```python
from build123d import *

# Parameters (mm, degrees)
SKETCH_1_W               = 20
SKETCH_1_H               = 20
SKETCH_1_R               = 2
SKETCH_1_R_2             = 2.15
EXTRUDE_1_DEPTH          = 46
CUT_EXTRUDE_1_REACH      = 50.125
PATTERN_CIRCULAR_1_COUNT = 4
FILLET_1_R               = 0.3
CUT_EXTRUDE_2_DEPTH      = 49.124837662
CUT_EXTRUDE_2_DEPTH_BACK = 49.124837662
SKETCH_2_R               = 2.5


with BuildPart() as part:
    # Sketch 1 → Extrude 1 (new body)
    with BuildSketch(Plane.XY):
        Rectangle(SKETCH_1_W, SKETCH_1_H)
        with Locations((-7, 7)):
            Circle(SKETCH_1_R, mode=Mode.SUBTRACT)
        with Locations((-7, -7)):
            Circle(SKETCH_1_R, mode=Mode.SUBTRACT)
        Circle(SKETCH_1_R_2, mode=Mode.SUBTRACT)
        with Locations((7, 7)):
            Circle(SKETCH_1_R, mode=Mode.SUBTRACT)
        with Locations((7, -7)):
            Circle(SKETCH_1_R, mode=Mode.SUBTRACT)
    extrude(amount=EXTRUDE_1_DEPTH)

    # Sketch 1_3 → Cut-Extrude 1 (cut, up to next)
    with BuildSketch(Plane.XY, mode=Mode.PRIVATE) as cut_extrude_1_sk1:
        with BuildLine():
            Line((-8.5, 2.65), (-10, 2.65))
            Line((-10, 2.65), (-10, -2.65))
            Line((-10, -2.65), (-8.5, -2.65))
            Line((-8.5, -2.65), (-8.5, -4.15))
            Line((-8.5, -4.15), (-4.503166667, -4.15))
            ThreePointArc((-4.503166667, -4.15), (-3.3, 0), (-4.503166667, 4.15))
            Line((-4.503166667, 4.15), (-8.5, 4.15))
            Line((-8.5, 4.15), (-8.5, 2.65))
        make_face()
    cut_extrude_1_tool1 = extrude(cut_extrude_1_sk1.sketch, amount=CUT_EXTRUDE_1_REACH, mode=Mode.PRIVATE) & part.part
    cut_extrude_1 = cut_extrude_1_tool1.solids().sort_by_distance((-6.606913, 0, 0))[0]
    add(cut_extrude_1, mode=Mode.SUBTRACT)

    # Pattern Circular 1: Cut-Extrude 1 ×4 about axis
    pattern_circular_1_axis = Axis((0, 0, 0), (0, 0, 1))
    for i in range(1, PATTERN_CIRCULAR_1_COUNT):
        add(cut_extrude_1.rotate(pattern_circular_1_axis, i * 360 / PATTERN_CIRCULAR_1_COUNT), mode=Mode.SUBTRACT)

    # Fillet 1
    fillet_1_edges = [part.edges().sort_by_distance(p)[0] for p in [
        (-10, -10, 23),
        (10, -10, 23),
        (10, 10, 23),
        (-10, 10, 23),
    ]]
    fillet(fillet_1_edges, radius=FILLET_1_R)

    # Sketch 2 → Cut-Extrude 2 (cut, two sides: drawn at the far end of the back side and taken through both)
    with BuildSketch(Plane(origin=(0, 0, 0), x_dir=(0, 0, -1), z_dir=(1, 0, 0)).offset(-CUT_EXTRUDE_2_DEPTH_BACK)):
        with Locations((-8.5, 0)):
            Circle(SKETCH_2_R)
    extrude(amount=CUT_EXTRUDE_2_DEPTH + CUT_EXTRUDE_2_DEPTH_BACK, mode=Mode.SUBTRACT)


solid = part.part
```
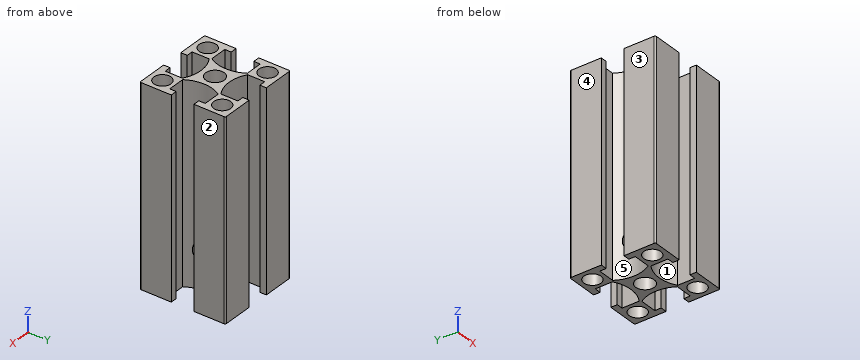
Here's how the part is built. I have some questions about the finished solid (model axes, mm). Face numbers are marked on the shaded views. A direction names the side the tool comes from. Coordinates: 2 decimals unless noted, no trailing zeros. Write each loop counter-clockwise with the first axis right and the second up, starting at its lowest first coordinate (ties: lowest second). Pieces come first, ordered by that corner, then holes. Notation, with made-up numbers: M -15,76.25 L 16,76.25 A23 ccw 16,110.25 Z; hole C -6,89 d7. An arc over 180 degrees is marked long. Answer as CSV lines item,"result". Start each with the question number.
Q1. I need wall thicknesses on probe 1 along Y at (x, z) = (-7, 33); probe 2 along X at (y, z) = (-6.5, 36); probe 3 along X at (y, z) = (-2.75, 9). Which ranges of each line are inside material? Lowest first, please. Write a range as [from, to].
Q2. Suppose I cut it at C-C, the plane z = 8.5. State how many separate pieces and enclosed holes the cut face has, then the cut area to 3 significant figures.
Q3. Suppose I cut it at A-A, the plane x = 7. List the corners of the cut face in (y, z) for me.
Q4. For the marked faces 4 and 5, which set-ups out of +Z, -Z, +X, -X, +Y, -Y let a thin tool reach every point of the face, with its end or its side?
Q5. Will these pins go through, and if not, where does the flat tip stop? pin 1 Ø1.5 at (x, z) = (-0.5, 8.5) entering from +Y; pin 2 Ø2.5 at (x, y) = (0, 0) entering from +Z.
Q6. If we mould it in two halves opening along X, with no side actions, what happens to the marked faces 1, 2 and 3? For each: pulls with the +X half, pulls with the -X half, needs draft (parallel to the pull), parting line crosses it, or undercut.
Q7. Suppose I cut it at D-D, the plane x = 0. List the corners of the cut face in (y, z) for me, then the cut area to 3 significant figures.
Entries:
1,probe 1,"y = [-10, -9], [-5, -4.15], [4.15, 5], [9, 10]"
1,probe 2,"x = [-10, -8.94], [-5.06, -4.15], [4.15, 5.06], [8.94, 10]"
1,probe 3,"x = [-10, -8.5], [-3.8, 3.8], [8.5, 10]"
2,separate pieces,"2"
2,enclosed holes,"4"
2,area,"124 mm²"
3,outline,"M -10,0 L -9,0 L -9,46 L -10,46 Z; M -5,0 L -4.15,0 L -4.15,46 L -5,46 Z; M 4.15,0 L 5,0 L 5,46 L 4.15,46 Z; M 9,0 L 10,0 L 10,46 L 9,46 Z"
4,face 4,"+Z, -Z, -X, +Y, -Y"
4,face 5,"+Z, -Z"
5,pin 1,"stops at y = 3.4"
5,pin 2,"passes through"
6,face 1,"undercut"
6,face 2,"pulls with the +X half"
6,face 3,"pulls with the -X half"
7,outline,"M -3.3,0 L -2.15,0 L -2.15,7.22 A2.5 cw -2.15,9.78 L -2.15,46 L -3.3,46 Z; M 2.15,0 L 3.3,0 L 3.3,46 L 2.15,46 L 2.15,9.78 A2.5 cw 2.15,7.22 Z"
7,area,"105 mm²"
